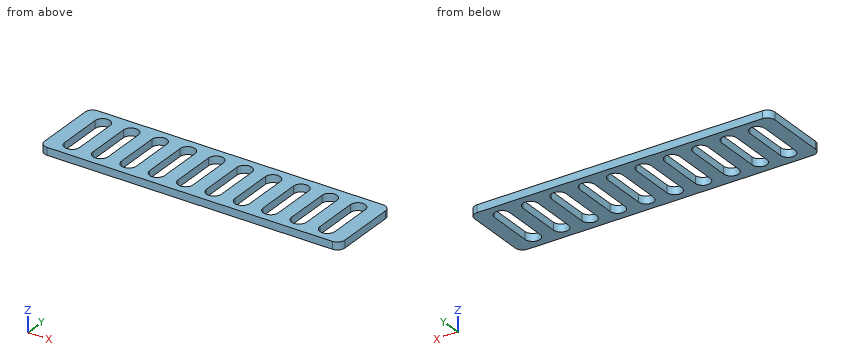
from build123d import *

# Parameters (mm, degrees)
PAD_DEPTH           = 5
POCKET_DEPTH        = 5
LINEARPATTERN_COUNT = 10
LINEARPATTERN_PITCH = 18.888889


with BuildPart() as part:
    # Sketch → Pad (new body)
    with BuildSketch(Plane.XY):
        with BuildLine():
            ThreePointArc((0, 5), (1.464466, 1.464466), (5, 0))
            Line((195, 0), (5, 0))
            ThreePointArc((195, 0), (198.535534, 1.464466), (200, 5))
            Line((200, 45), (200, 5))
            ThreePointArc((200, 45), (198.535534, 48.535534), (195, 50))
            Line((5, 50), (195, 50))
            ThreePointArc((5, 50), (1.464466, 48.535534), (0, 45))
            Line((0, 5), (0, 45))
        make_face()
    extrude(amount=PAD_DEPTH)

    # Sketch001 (on Face10 of Pad) → Pocket (cut)
    with BuildSketch(Plane.XY.offset(5)):
        with BuildLine():
            ThreePointArc((10, 10), (15, 5), (20, 10))
            Line((20, 10), (20, 40))
            ThreePointArc((20, 40), (15, 45), (10, 40))
            Line((10, 40), (10, 10))
        make_face()
    pocket = extrude(amount=-POCKET_DEPTH, mode=Mode.SUBTRACT)

    # LinearPattern: Pocket ×10
    with Locations(*[(i * LINEARPATTERN_PITCH, 0, 0) for i in range(1, LINEARPATTERN_COUNT)]):
        add(pocket, mode=Mode.SUBTRACT)


solid = part.part
Verification items for the finished model (mm, model axes). Round coordinates to 2 decimals unless told otherwise and drop trailing zeros. Loops run counter-clockwise (first coordinate to the right, second up) from the corner with the lowest first, then second, coordinate; pieces in that order, holes last. Notation, with made-up numbers: (1.25, 71) - (35.25, 71) arc R34 ccw to (35.25, 109) - close; hole circle Ø6 at (20, 80.25). An arc over 180 degrees is marked (long way). Use a Markdown table: item, result. Add a question column.
1. Section check B-B, the plane y = 23. Give the number of separate pieces and of enclosed holes in the cut face, plus the area to 3 significant figures.
2. Thickness scan on probe 1 along Y at (x, z) = (162, 0.6); probe 2 along Y at (x, z) = (13, 2.3); probe 3 along X at (y, z) = (46.5, 1.9). Record the ranges inside material, lowest first. Write a range as [from, to].
3. Section check A-A, the plane x = 15. Record the boundary of the cut face in (y, z).
4. Section check D-D, the plane x = 88.5. Record the boundary of the cut face in (y, z), plus the area to 3 significant figures.
Checks:
| question | item | result |
|---|---|---|
| 1 | separate pieces | 11 |
| 1 | enclosed holes | 0 |
| 1 | area | 500 mm^2 |
| 2 | probe 1 | y = [0, 7.15], [42.85, 50] |
| 2 | probe 2 | y = [0, 5.42], [44.58, 50] |
| 2 | probe 3 | x = [0.23, 199.77] |
| 3 | outline | (0, 0) - (5, 0) - (5, 5) - (0, 5) - close; (45, 0) - (50, 0) - (50, 5) - (45, 5) - close |
| 4 | outline | (0, 0) - (5.44, 0) - (5.44, 5) - (0, 5) - close; (44.56, 0) - (50, 0) - (50, 5) - (44.56, 5) - close |
| 4 | area | 54.4 mm^2 |
